CAD build for the part. Positions are in the model's coordinates, mm. Give positions to 0.01 mm unless a question says otherwise; leave off trailing zeros. Write each loop counter-clockwise with the first axis right and the second up, starting at its lowest first coordinate (ties: lowest second). Pieces come first, ordered by that corner, then holes. Notation, with made-up numbers: (45, 88) - (61, 88) arc R20 cw to (61, 111) - close; hole circle Ø11 at (53, 61). An arc over 180 degrees is marked (long way). Put each result on its own line as item: value. Start each with the question number.
1. Cut at B-B on z = 3.5. List the corners of the cut face in (x, y), and give its area (3 significant figures).
2. Mould opens along Z. For faces 1 (the cylindrical face through (-0.22, 0.99, 7)), 2 (the flat face through (0, 0, 0)), 3 (the flat face through (0, 0, 10.317)) say: +Z half, -Z half, draft (parallel to the pull), parting line (faces both ways), or undercut.
3. Cut at A-A on z = 7.75. List the corners of the cut face in (x, y), and give its area (3 significant figures).
4. Wall check: line 1 (X direction, y = -0.75, z = 8.5); line 2 (Y direction, x = -1.75, z = 2.25); line 3 (Y direction, x = -2, z = 1.5). Give the ranges that are in metal, low to high.
from build123d import *

# Parameters (mm, degrees)
FILLET1_R = 0.254


with BuildPart() as part:
    # Sketch1 → Revolve1 (revolve)
    with BuildSketch(Plane(origin=(0, 0, 0), x_dir=(1, 0, 0), z_dir=(0, 1, 0))):
        Polygon((0, 0), (3.048, 0), (3.048, -2.54), (1.016, -3.713175747), (1.016, -10.317175747), (0, -10.317175747), align=None)
    revolve(axis=Axis((0, 0, 10.317175747), (0, 0, -1)))

    # Fillet1
    fillet1_edges = [part.edges().sort_by_distance(p)[0] for p in [
        (-1.016, 0, 10.317175747),
        (-1.016, 0, 3.713175747),
        (-3.048, 0, 2.54),
        (-3.048, 0, 0),
    ]]
    fillet(fillet1_edges, radius=FILLET1_R)


solid = part.part
Report:
1. outline: circle Ø2.77 at (0, 0)
1. area: 6.03 mm²
2. face 1: draft
2. face 2: -Z half
2. face 3: +Z half
3. outline: circle Ø2.03 at (0, 0)
3. area: 3.24 mm²
4. line 1: x = -0.69 to 0.69
4. line 2: y = -2.5 to 2.5
4. line 3: y = -2.3 to 2.3
